Source: three-view drawing plus pictorial views. Frame: mm from the lowest corner of the part. A direction names the side the tool comes from. Give positions to 0.01 mm unless a question says otherwise; leave off trailing zeros. Order: outer loops, then holes, each group sorted by start corner. A loop starts at its lowest first (then second) coordinate and runs counter-clockwise, first axis right, second up. Notation, with made-up numbers: M -38.5,-27.5 L -12.5,-27.5 A16 ccw -12.5,-8.5 Z; hole C 0.25,79.5 d6. An arc over 180 degrees is marked long. Use CSV: the item, a comma, the result in double quotes.
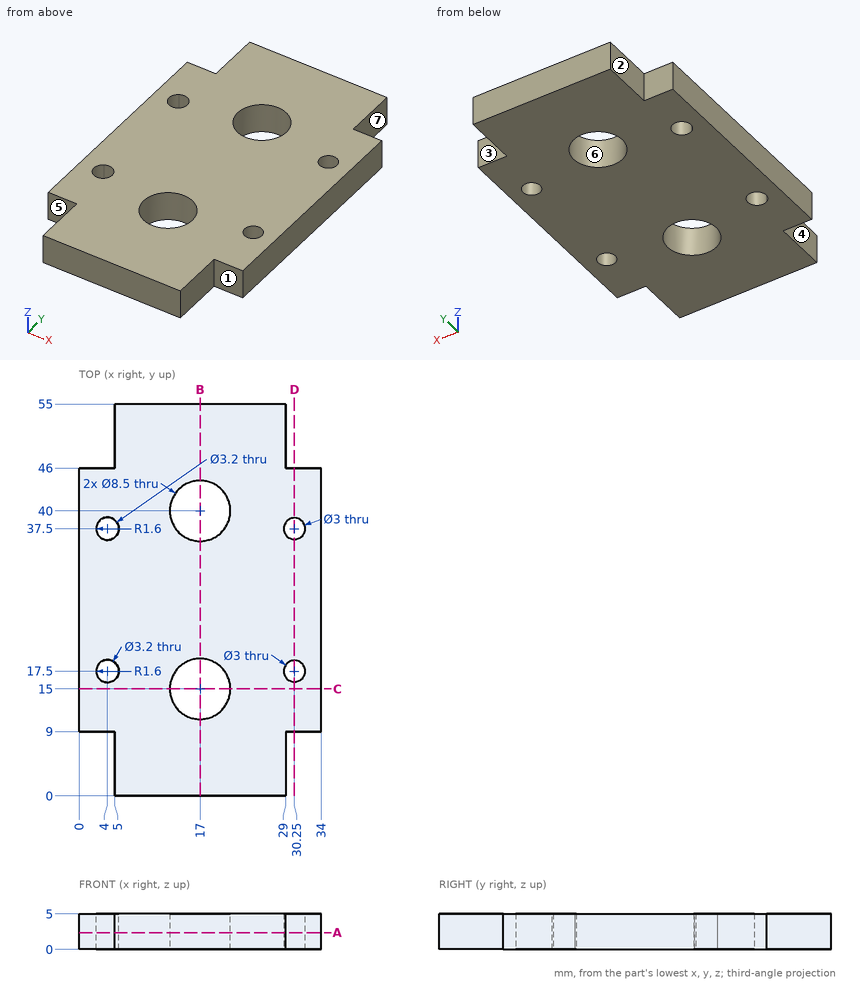
1. Pin query (flat end, axial travel): pin 1 Ø5 at (x, y) = (17, 40) entering from +Z; pin 2 Ø1.5 at (y, z) = (52.5, 2) entering from +X; pin 3 Ø2.5 at (x, z) = (30.5, 3.5) entering from -Y; pin 4 Ø1.5 at (x, z) = (32.5, 1.5) entering from +Y. Return the tip coordinate at first contact, or that it passes through.
Answer:
pin 1,"through"
pin 2,"x = 29"
pin 3,"y = 9"
pin 4,"y = 46"
2. Pull-direction query (X, two-part tool) for the marked faces 5, 6 and 7; classes: +X half, -X half, draft (parallel to the pull), parting line (faces both ways), or undercut.
Answer:
face 5,"draft"
face 6,"undercut"
face 7,"+X half"
3. Line query: line 1 (Y direction, x = 4, z = 1.75); line 2 (Y direction, x = 18, z = 0.9); line 3 (X direction, y = 18, z = 1.65). Output: solid intervals per line, ascending.
Answer:
line 1,"9 to 15.9, 19.1 to 35.9, 39.1 to 46"
line 2,"0 to 10.87, 19.13 to 35.87, 44.13 to 55"
line 3,"0 to 2.48, 5.52 to 13.99, 20.01 to 28.84, 31.66 to 34"
4. Section B-B, the plane x = 17. Return the cut outline in (y, z), plus the area to 3 significant figures.
Answer:
outline,"M 0,0 L 10.75,0 L 10.75,5 L 0,5 Z; M 19.25,0 L 35.75,0 L 35.75,5 L 19.25,5 Z; M 44.25,0 L 55,0 L 55,5 L 44.25,5 Z"
area,"190 mm2"
5. Section A-A, the plane z = 2.35. Return the cut outline in (x, y), plus the area to 3 significant figures.
Answer:
outline,"M 0,9 L 5,9 L 5,0 L 29,0 L 29,9 L 34,9 L 34,46 L 29,46 L 29,55 L 5,55 L 5,46 L 0,46 Z; hole C 4,17.5 d3.2; hole C 4,37.5 d3.2; hole C 17,15 d8.5; hole C 17,40 d8.5; hole C 30.25,17.5 d3; hole C 30.25,37.5 d3"
area,"1,550 mm2"
6. Section C-C, the plane y = 15. Return the cut outline in (x, z), plus the area to 4 significant figures.
Answer:
outline,"M 0,0 L 12.75,0 L 12.75,5 L 0,5 Z; M 21.25,0 L 34,0 L 34,5 L 21.25,5 Z"
area,"127.5 mm2"
7. Section D-D, the plane x = 30.25. Return the cut outline in (y, z), plus the area to 3 significant figures.
Answer:
outline,"M 9,0 L 16,0 L 16,5 L 9,5 Z; M 19,0 L 36,0 L 36,5 L 19,5 Z; M 39,0 L 46,0 L 46,5 L 39,5 Z"
area,"155 mm2"
8. Reachability of the marked faces 1, 2, 3 and 4 from +Z, -Z, +X, -X, +Y, -Y: full face, straight path, thin tool, end or side. Return the list, or none.
Answer:
face 1,"+Z, -Z, +X, -Y"
face 2,"+Z, -Z, -X, +Y"
face 3,"+Z, -Z, +X, +Y"
face 4,"+Z, -Z, -X, -Y"
